Study the drawing (mm; zero at the part's minimum x, y, z) and answer. Round coordinates to 2 decimals unless told otherwise and drop trailing zeros. Write each loop counter-clockwise with the first axis right and the second up, starting at its lowest first coordinate (ties: lowest second). Pieces come first, ordered by that corner, then holes. Notation, with made-up numbers: (-3, -0.75) - (11, -0.75) arc R17 ccw to (11, 14.25) - close; hole circle Ø1 at (18.25, 2). An arc over 180 degrees is marked (long way). Use one line per item in the form item = value. Start each with the question number.
1) The part is cut by section D-D, the plane z = 65. Give the vertices of the cut face in (x, y) (1 decimal).
2) For a pull along X with two mould halves and no side action, classify the marked faces 1 and 2 as released by +X, released by -X, zero draft, split by the parting line, or undercut.
3) The part is cut by section C-C, the plane x = 399. Give the vertices of the cut face in (y, z) (3 decimals), plus the area to 3 significant figures.
4) Consider line 1 along X through (y, z) = (29.5, 300); line 2 along Z through (x, y) = (466, 74); line 3 along X through (y, z) = (95.5, 97). Determine where each line is inside the solid, lowest interval first. Write a range as from..to.
5) This flat-tipped pin is pushed along its axis until it touches: pin 1 (2 mm diameter, centred on x = 702.5, y = 51.5, fed in from +Z). Where does it stop, or does it pass through?
6) The part is cut by section A-A, the plane z = 233. Give the vertices of the cut face in (x, y) (3 decimals), plus the area to 3 significant figures.
7) The part is cut by section B-B, the plane y = 79. Give the vertices of the cut face in (x, z), plus the area to 3 significant figures.
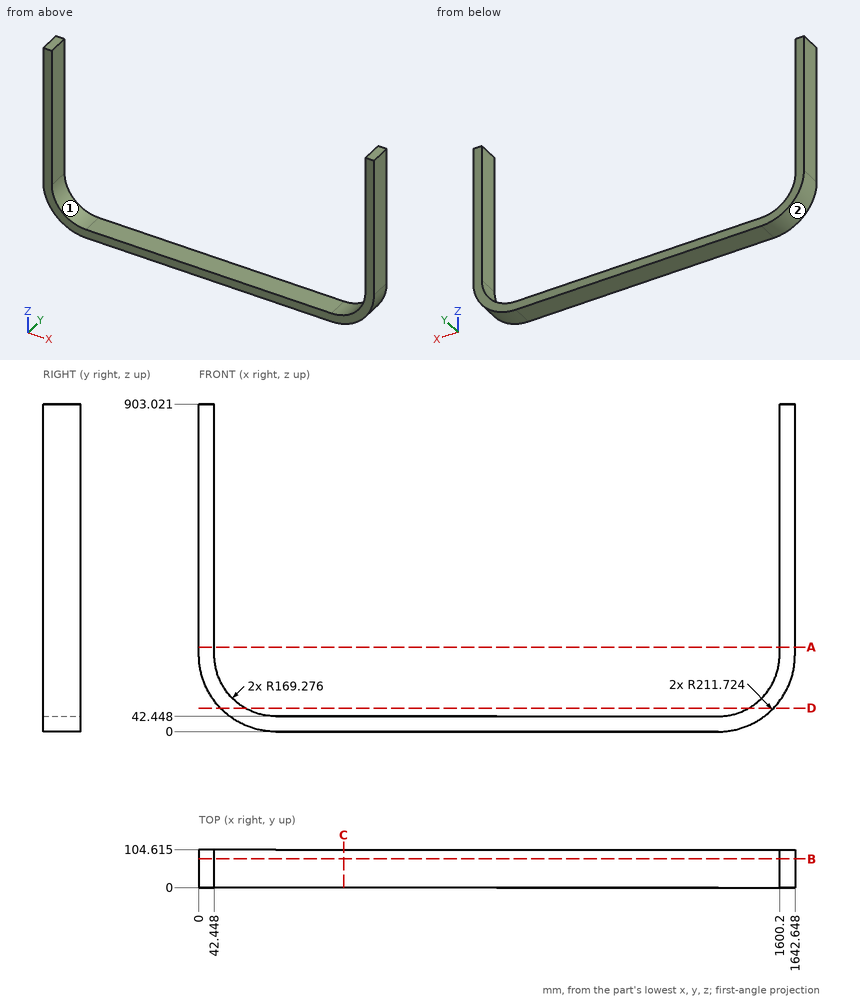
Geometry results:
q1.outline = (59.1, 0) - (127.3, 0) - (127.3, 104.6) - (59.1, 104.6) - close; (1515.3, 0) - (1583.6, 0) - (1583.6, 104.6) - (1515.3, 104.6) - close
q2.face_1 = undercut
q2.face_2 = released by -X
q3.outline = (0, 0) - (104.615, 0) - (104.615, 42.448) - (0, 42.448) - close
q3.area = 4,440 mm2
q4.line_1 = 0..42.45, 1600.2..1642.65
q4.line_2 = 0..42.45
q4.line_3 = 33.78..87.25, 1555.39..1608.87
q5.pin_1 = 42.45
q6.outline = (0, 0) - (42.448, 0) - (42.448, 104.615) - (0, 104.615) - close; (1600.2, 0) - (1642.648, 0) - (1642.648, 104.615) - (1600.2, 104.615) - close
q6.area = 8,880 mm2
q7.outline = (0, 211.72) arc R211.72 ccw to (211.72, 0) - (1430.92, 0) arc R211.72 ccw to (1642.65, 211.72) - (1642.65, 903.02) - (1600.2, 903.02) - (1600.2, 211.72) arc R169.28 cw to (1430.92, 42.45) - (211.72, 42.45) arc R169.28 cw to (42.45, 211.72) - (42.45, 903.02) - (0, 903.02) - close
q7.area = 136,000 mm2
